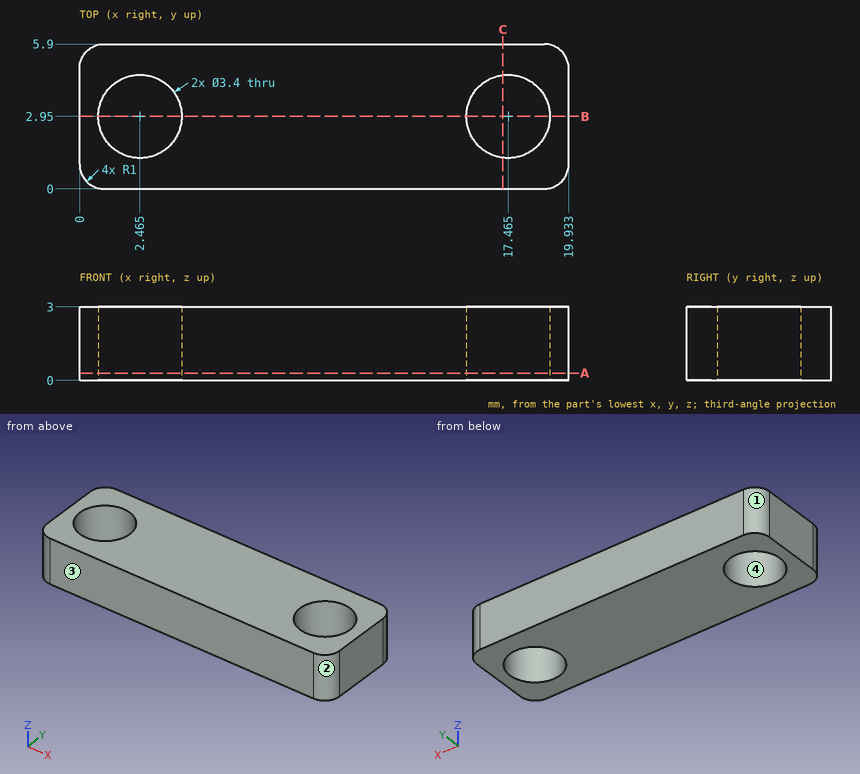
Source: three-view drawing plus pictorial views. Frame: mm from the lowest corner of the part. Give positions to 0.01 mm unless a question says otherwise; leave off trailing zeros. Order: outer loops, then holes, each group sorted by start corner. A loop starts at its lowest first (then second) coordinate and runs counter-clockwise, first axis right, second up. Notation, with made-up numbers: (-10.75, 61) -> (29.25, 61) arc R24 cw to (29.25, 76) -> close; hole circle Ø2 at (14.25, -27.75). An arc over 180 degrees is marked (long way). Use a Markdown table: item, result.
Q1. Material intervals for line 1 (X direction, y = 4.3, z = 1.6) (1 decimal); line 2 (X direction, y = 2.65, z = 1.3); line 3 (Y direction, x = 1.5, z = 0.55), sorted ascending. Write a range as [from, to].
A:
| item | result |
|---|---|
| line 1 | [0, 1.4], [3.5, 16.4], [18.5, 19.9] |
| line 2 | [0, 0.79], [4.14, 15.79], [19.14, 19.93] |
| line 3 | [0, 1.55], [4.35, 5.9] |
Q2. Pull-direction query (X, two-part tool) for the marked faces 1, 2, 3 and 4; classes: +X half, -X half, draft (parallel to the pull), parting line (faces both ways), or undercut.
A:
| item | result |
|---|---|
| face 1 | -X half |
| face 2 | +X half |
| face 3 | draft |
| face 4 | undercut |
Q3. Section C-C (x = 17.25). Return the cut outline in (y, z).
A:
| item | result |
|---|---|
| outline | (0, 0) -> (1.26, 0) -> (1.26, 3) -> (0, 3) -> close; (4.64, 0) -> (5.9, 0) -> (5.9, 3) -> (4.64, 3) -> close |
Q4. Section B-B (y = 2.95). Return the cut outline in (x, z) (1 decimal).
A:
| item | result |
|---|---|
| outline | (0, 0) -> (0.8, 0) -> (0.8, 3) -> (0, 3) -> close; (4.2, 0) -> (15.8, 0) -> (15.8, 3) -> (4.2, 3) -> close; (19.2, 0) -> (19.9, 0) -> (19.9, 3) -> (19.2, 3) -> close |
Q5. Section A-A (z = 0.3). State how many separate pieces and enclosed holes the cut face has.
A:
| item | result |
|---|---|
| separate pieces | 1 |
| enclosed holes | 2 |
Q6. First-contact query: P1, Ø2, axis at x = 17.465, y = 2.95, coming from the -Z side; P2, Ø1.5, axis at y = 4, z = 2.5, coming from the -X side. Flat tips, straight axial feed; report the tip coordinate or a pass-through.
A:
| item | result |
|---|---|
| P1 | through |
| P2 | x = 0 |
